from build123d import *

# Parameters (mm, degrees)
F1_DEPTH = 3.175
F2_R     = 5.08


with BuildPart() as f1:
    # F0 (on Top) → F1 (new body, symmetric)
    with BuildSketch(Plane.XY):
        Polygon((327.903505, 0), (-307.096495, 0), (-256.296495, -50.8), (277.103505, -50.8), align=None)
    extrude(amount=F1_DEPTH, both=True)

    # F2
    f2_edges = [f1.edges().sort_by_distance(p)[0] for p in [
        (10.403505, 0, -3.175),
        (10.403505, -50.8, -3.175),
    ]]
    fillet(f2_edges, radius=F2_R)


solid = f1.part
Geometry: final body of the model. Coordinates: model frame, mm. Round coordinates to 2 decimals unless told otherwise and drop trailing zeros. Loops run counter-clockwise (first coordinate to the right, second up) from the corner with the lowest first, then second, coordinate; pieces in that order, holes last. Notation, with made-up numbers: (57.25, -21) -> (111.25, -21) arc R17 ccw to (111.25, 3) -> close; hole circle Ø9 at (12.5, -36.5). An arc over 180 degrees is marked (long way). One line per question, with ' | ' between items. Start each with the question number.
1. Section C-C on z = 0.5. Output: boundary loops of the cut face in (x, y), and give its area (3 significant figures).
2. Section B-B on y = -22. Output: boundary loops of the cut face in (x, z) (1 decimal), and give its area (3 significant figures).
3. Line query: line 1 along Y through (x, z) = (-179.5, 1); line 2 along Y through (x, z) = (103, 1.75); line 3 along Z through (x, y) = (-9, -47.5) (3 decimals). Output: solid intervals per line, ascending. Write a range as [from, to].
4. Section A-A on x = 157.5. Output: boundary loops of the cut face in (y, z) (3 decimals), and give its area (3 significant figures).
5. Contact query for flat-ended pins moving along their axis: pin 1 (1.5 mm diameter, centred on y = -10, z = 1, fed in from -X); pin 2 (2 mm diameter, centred on x = -49, z = 1.5, fed in from +Y). Output: stop coordinate, or through.
Returned:
1) outline: (-306.9, -0.2) -> (-256.49, -50.6) -> (277.3, -50.6) -> (327.71, -0.2) -> close | area: 29,400 mm2
2) outline: (-285.1, -3.2) -> (305.9, -3.2) -> (305.9, 3.2) -> (-285.1, 3.2) -> close | area: 3,750 mm2
3) line 1: y = [-50.72, -0.08] | line 2: y = [-50.8, 0] | line 3: z = [-2.853, 3.175]
4) outline: (-50.8, 1.905) arc R5.08 ccw to (-45.72, -3.175) -> (-5.08, -3.175) arc R5.08 ccw to (0, 1.905) -> (0, 3.175) -> (-50.8, 3.175) -> close | area: 312 mm2
5) pin 1: stops at x = -297.85 | pin 2: stops at y = 0
